from build123d import *

# Parameters (mm, degrees)
BOSS_EXTRU_2_DEPTH      = 2
ESQUISSE2_W             = 20
ESQUISSE2_H             = 2
BOSS_EXTRU_3_DEPTH      = 20.55
ESQUISSE3_W             = 20
ESQUISSE3_H             = 2
BOSS_EXTRU_4_DEPTH      = 4
ESQUISSE4_R             = 1.5
ENL_V_MAT_EXTRU_1_DEPTH = 4


with BuildPart() as part:
    # Esquisse1 → Boss.-Extru.2 (new body)
    with BuildSketch(Plane.XY):
        with BuildLine():
            Line((-10, 2.5), (-10, -2.5))
            Line((-10, -2.5), (-7.538516481, -2.5))
            ThreePointArc((-7.538516481, -2.5), (-7.849183513, 0.136481848), (-5.5, -1.1))
            ThreePointArc((-5.5, -1.1), (-5.763518152, -1.949183513), (-6.461483519, -2.5))
            Line((-6.461483519, -2.5), (6.461483519, -2.5))
            ThreePointArc((6.461483519, -2.5), (6.150816487, 0.136481848), (8.5, -1.1))
            ThreePointArc((8.5, -1.1), (8.236481848, -1.949183513), (7.538516481, -2.5))
            Line((7.538516481, -2.5), (10, -2.5))
            Line((10, -2.5), (10, 2.5))
            Line((10, 2.5), (-10, 2.5))
        make_face()
    extrude(amount=BOSS_EXTRU_2_DEPTH)

    # Esquisse2 → Boss.-Extru.3 (add)
    with BuildSketch(Plane.XY.offset(2)):
        with Locations((0, 1.5)):
            Rectangle(ESQUISSE2_W, ESQUISSE2_H)
    extrude(amount=BOSS_EXTRU_3_DEPTH)

    # Esquisse3 → Boss.-Extru.4 (add)
    with BuildSketch(Plane(origin=(0, 2.5, 0), x_dir=(1, 0, 0), z_dir=(0, 1, 0))):
        with Locations((0, -21.55)):
            Rectangle(ESQUISSE3_W, ESQUISSE3_H)
    extrude(amount=BOSS_EXTRU_4_DEPTH)

    # Esquisse4 → Enlèv. mat.-Extru.1 (cut)
    with BuildSketch(Plane.XY.offset(22.55)):
        with Locations((0.45, 4)):
            Circle(ESQUISSE4_R)
    extrude(amount=-ENL_V_MAT_EXTRU_1_DEPTH, mode=Mode.SUBTRACT)


solid = part.part
Source: CAD feature listing. Evaluate the final solid. Frame: model axes, mm. A direction names the side the tool comes from. Round coordinates to 2 decimals unless told otherwise and drop trailing zeros. Write each loop counter-clockwise with the first axis right and the second up, starting at its lowest first coordinate (ties: lowest second). Pieces come first, ordered by that corner, then holes. Notation, with made-up numbers: M 19,82.25 L 78,82.25 A22 ccw 78,111.25 Z; hole C 51,23 d6. An arc over 180 degrees is marked long. One line per item, written item: value. Start each with the question number.
Item 1: Ray query, L1, parallel to X at y = -1.1, z = 0.6; L2, parallel to Y at x = 0.45, z = 21.9; L3, parallel to Y at x = 5.75, z = 11.5. Return the intervals inside material, ascending. Write a range as from..to.
Item 2: Section query C-C (z = 9). Return the cut outline in (x, y), plus the area to 3 significant figures.
Item 3: Section query A-A (y = 4). Return the cut outline in (x, z).
Item 4: Section query B-B (x = 7). Return the cut outline in (y, z), plus the area to 3 significant figures.
Item 5: Mould query, pull axis X, two halves, no side actions, for faces 4 (the flat face through (10, 2, 11)), 5 (the flat face through (-10, 2, 11)), 6 (the flat face through (0, 2.5, 10)), 7 (the cylindrical face through (1.256, 5.265, 21.564)). Classes: pulls with the +X half, pulls with the -X half, needs draft (parallel to the pull), parting line crosses it, or undercut.
Item 6: Set-up query: faces 1 (the flat face through (0, 6.5, 22)), 2 (the flat face through (0, -1, 2)), 3 (the flat face through (0, 6, 20.55)). Return all of +Z, -Z, +X, -X, +Y, -Y with unobstructed straight access to the full face (end or side cutting, diameter ignored); none if empty.
Item 7: Pin query (flat end, axial travel): pin 1 (3 mm diameter, centred on x = 4, z = 7, fed in from +Y); pin 2 (1.2 mm diameter, centred on x = 1.5, y = 5, fed in from -Z); pin 3 (4 mm diameter, centred on x = 1.5, z = 3, fed in from -Y); pin 4 (2.5 mm diameter, centred on x = -4, y = -1, fed in from +Z). Return the tip coordinate at first contact, or that it passes through.
Result set:
1. L1: x = -10..-8.5, -5.5..5.5, 8.5..10
1. L2: y = 0.5..2.5, 5.5..6.5
1. L3: y = 0.5..2.5
2. outline: M -10,0.5 L 10,0.5 L 10,2.5 L -10,2.5 Z
2. area: 40.0 mm²
3. outline: M -10,20.55 L -1.05,20.55 L -1.05,22.55 L -10,22.55 Z; M 1.95,20.55 L 10,20.55 L 10,22.55 L 1.95,22.55 Z
4. outline: M 0.4,0 L 2.5,0 L 2.5,20.55 L 6.5,20.55 L 6.5,22.55 L 0.5,22.55 L 0.5,2 L 0.4,2 Z
4. area: 53.3 mm²
5. face 4: pulls with the +X half
5. face 5: pulls with the -X half
5. face 6: needs draft
5. face 7: undercut
6. face 1: +Z, -Z, +X, -X, +Y
6. face 2: +Z, +X, -X, -Y
6. face 3: -Z, +X, -X, +Y
7. pin 1: stops at y = 2.5
7. pin 2: stops at z = 20.55
7. pin 3: stops at y = -2.5
7. pin 4: stops at z = 2
